CAD build for the part. Positions are in the model's coordinates, mm. Face numbers are marked on the shaded views. A direction names the side the tool comes from. Coordinates: 2 decimals unless noted, no trailing zeros. Write each loop counter-clockwise with the first axis right and the second up, starting at its lowest first coordinate (ties: lowest second). Pieces come first, ordered by that corner, then holes. Notation, with made-up numbers: (-36.5, 83) - (5.5, 83) arc R11 ccw to (5.5, 98) - close; hole circle Ø3 at (57, 23.25). An arc over 180 degrees is marked (long way). One line per question, with ' | ' between items. Start each with the question number.
1. Band-saw the part on A-A, the plane y = 0. Write the cut outline in (x, z), then the cut area to 3 significant figures.
2. Which spindle directions (+Z, -Z, +X, -X, +Y, -Y) get a long thin tool onto all of the face, cutting with end or side? Do the marked faces 1 and 2. Say none if no direction does.
3. Flat gauge pins, fed straight in: P1, Ø1.5, axis at x = 4.5, y = 6, coming from the -Z side; P2, Ø1.5, axis at x = 1, y = 7.5, coming from the +Z side; P3, Ø3, axis at x = 4.5, z = -8.5, coming from the -Y side; P4, Ø1.9, axis at y = 0, z = 0, coming from the +X side. Where does each tip first touch, or does it go through?
4. Band-saw the part on D-D, the plane z = 5.75. Write the cut outline in (x, y), then the cut area to 3 significant figures.
5. Band-saw the part on C-C, the plane y = -3. Write the cut outline in (x, z), then the cut area to 3 significant figures.
6. Probe line 1 (Y direction, x = 3.7, z = 0); line 2 (Z direction, x = 0.45, y = 1); line 3 (X direction, y = -8, z = 9.5). List the from-to ranges inside material, lowest first.
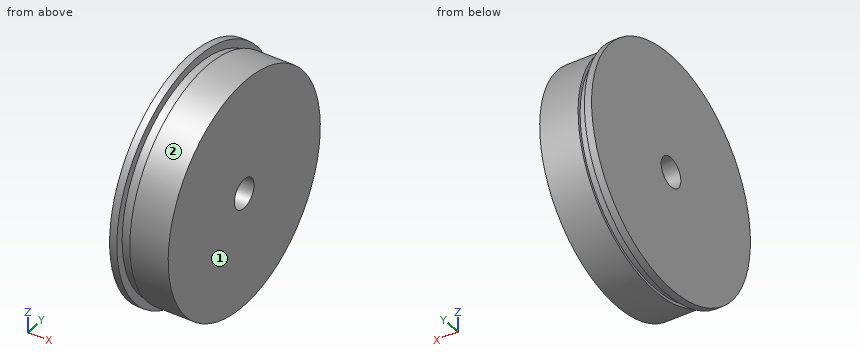
from build123d import *

# Parameters (mm, degrees)
SKETCH3_R          = 1.5748
CUT_EXTRUDE1_DEPTH = 19.886740428


with BuildPart() as part:
    # Sketch2 → Revolve1 (revolve)
    with BuildSketch(Plane.XY, mode=Mode.PRIVATE) as revolve1_sk:
        Polygon((0, 0), (0, -12.7), (0.762, -12.7), (0.762, -11.8491), (1.778, -11.8491), (1.778, -12.1666), (5.842, -12.1666), (5.842, 0), align=None)
    revolve(revolve1_sk.sketch.rotate(Axis((0, 0, 0), (1, 0, 0)), 270), axis=Axis((0, 0, 0), (1, 0, 0)))

    # Sketch3 → Cut-Extrude1 (cut, through all)
    with BuildSketch(Plane(origin=(5.842, 0, 0), x_dir=(0, 0, -1), z_dir=(1, 0, 0))):
        Circle(SKETCH3_R)
    extrude(amount=-CUT_EXTRUDE1_DEPTH, mode=Mode.SUBTRACT)


solid = part.part
Filled in:
1) outline: (0, -12.7) - (0.76, -12.7) - (0.76, -11.85) - (1.78, -11.85) - (1.78, -12.17) - (5.84, -12.17) - (5.84, -1.57) - (0, -1.57) - close; (0, 1.57) - (5.84, 1.57) - (5.84, 12.17) - (1.78, 12.17) - (1.78, 11.85) - (0.76, 11.85) - (0.76, 12.7) - (0, 12.7) - close | area: 124 mm²
2) face 1: +Z, -Z, +X, +Y, -Y | face 2: +X
3) P1: stops at z = -10.98 | P2: stops at z = 10.73 | P3: stops at y = -9.95 | P4: passes through
4) outline: (0, -11.32) - (0.76, -11.32) - (0.76, -10.36) - (1.78, -10.36) - (1.78, -10.72) - (5.84, -10.72) - (5.84, 10.72) - (1.78, 10.72) - (1.78, 10.36) - (0.76, 10.36) - (0.76, 11.32) - (0, 11.32) - close | area: 125 mm²
5) outline: (0, -12.34) - (0.76, -12.34) - (0.76, -11.46) - (1.78, -11.46) - (1.78, -11.79) - (5.84, -11.79) - (5.84, 11.79) - (1.78, 11.79) - (1.78, 11.46) - (0.76, 11.46) - (0.76, 12.34) - (0, 12.34) - close | area: 138 mm²
6) line 1: y = -12.17 to -1.57, 1.57 to 12.17 | line 2: z = -12.66 to -1.22, 1.22 to 12.66 | line 3: x = 0 to 0.76
